from build123d import *

# Parameters (mm, degrees)
F0_W     = 96
F0_H     = 26
F0_R     = 4
F1_DEPTH = 2
F5_W     = 96
F5_H     = 26
F5_R     = 4
F6_DEPTH = 2
F4_W     = 96
F4_H     = 26
F4_R     = 4
F7_DEPTH = 2
F8_R     = 2


with BuildPart() as f1:
    # F0 (on Top) → F1 (new body)
    with BuildSketch(Plane.XY):
        with Locations((17.3164154523, 0.965568237)):
            Rectangle(F0_W, F0_H)
        with Locations((17.3164154523, 0.965568237)):
            Circle(F0_R, mode=Mode.SUBTRACT)
        with Locations((-18.6835845477, 0.965568237)):
            Circle(F0_R, mode=Mode.SUBTRACT)
        with Locations((53.3164154523, 0.965568237)):
            Circle(F0_R, mode=Mode.SUBTRACT)
    extrude(amount=F1_DEPTH)

    # F5 (on offset) → F6 (join)
    with BuildSketch(Plane.XZ.offset(12.034431763)):
        with Locations((17.3164154523, -11)):
            Rectangle(F5_W, F5_H)
        with Locations((-18.6835845477, -11)):
            Circle(F5_R, mode=Mode.SUBTRACT)
        with Locations((17.3164154523, -11)):
            Circle(F5_R, mode=Mode.SUBTRACT)
        with Locations((53.3164154523, -11)):
            Circle(F5_R, mode=Mode.SUBTRACT)
    extrude(amount=F6_DEPTH)

    # F4 (on offset) → F7 (join)
    with BuildSketch(Plane(origin=(0, 13.965568237, 0), x_dir=(-1, 0, 0), z_dir=(0, 1, 0))):
        with Locations((-17.3164154523, -11)):
            Rectangle(F4_W, F4_H)
        with Locations((-53.3164154523, -11)):
            Circle(F4_R, mode=Mode.SUBTRACT)
        with Locations((-17.3164154523, -11)):
            Circle(F4_R, mode=Mode.SUBTRACT)
        with Locations((18.6835845477, -11)):
            Circle(F4_R, mode=Mode.SUBTRACT)
    extrude(amount=F7_DEPTH)

    # F8
    f8_edges = [f1.edges().sort_by_distance(p)[0] for p in [
        (17.316415, -14.034432, 2),
        (17.316415, 15.965568, 2),
        (65.316415, 14.965568, -24),
        (65.316415, -13.034432, -24),
        (-30.683585, 14.965568, -24),
        (-30.683585, -13.034432, -24),
    ]]
    fillet(f8_edges, radius=F8_R)


solid = f1.part
Could you check a few things on this model? Use its own coordinates, in mm. A direction names the side the tool comes from. Round coordinates to 2 decimals unless told otherwise and drop trailing zeros. Write each loop counter-clockwise with the first axis right and the second up, starting at its lowest first coordinate (ties: lowest second). Pieces come first, ordered by that corner, then holes. Notation, with made-up numbers: (54.5, -4) -> (65.5, -4) arc R15 cw to (65.5, 6) -> close; hole circle Ø11 at (-39.5, -11). An arc over 180 degrees is marked (long way). Use a Markdown table: item, result.
1. If we section it at C-C (x = 15.5): List the corners of the cut face in (y, z) for me.
Answer key:
| item | result |
|---|---|
| outline | (-14.03, -24) -> (-12.03, -24) -> (-12.03, -14.56) -> (-14.03, -14.56) -> close; (-14.03, -7.44) -> (-12.03, -7.44) -> (-12.03, 0) -> (-2.6, 0) -> (-2.6, 2) -> (-12.03, 2) arc R2 ccw to (-14.03, 0) -> close; (4.53, 0) -> (13.97, 0) -> (13.97, -7.44) -> (15.97, -7.44) -> (15.97, 0) arc R2 ccw to (13.97, 2) -> (4.53, 2) -> close; (13.97, -24) -> (15.97, -24) -> (15.97, -14.56) -> (13.97, -14.56) -> close |
2. Which directions (+Z, -Z, +X, -X, +Y, -Y) give clear straight access to the entire face, cutting with the end or side of a thin tool? Please do faces 4 (the face through (17, -12.034, -17)), 5 (the face through (-17.8, 15, -14.9)).
Answer key:
| item | result |
|---|---|
| face 4 | -Z, +X, -X |
| face 5 | +Y, -Y |
3. If we section it at D-D (y = -4.75): List the corners of the cut face in (x, z) for me.
Answer key:
| item | result |
|---|---|
| outline | (-30.68, 0) -> (65.32, 0) -> (65.32, 2) -> (-30.68, 2) -> close |
4. For pin 1 Ø1.5 at (x, y) = (33.5, 6) entering from -Z; pin 2 Ø5 at (x, z) = (53.32, -11) entering from +Y, each with a flat end and sliding along its axis, tell me the tip position at first contact or that it passes through.
Answer key:
| item | result |
|---|---|
| pin 1 | stops at z = 0 |
| pin 2 | passes through |
5. If we section it at B-B (z = -11): State how many separate pieces and enclosed holes the cut face has, then the cut area to 3 significant figures.
Answer key:
| item | result |
|---|---|
| separate pieces | 8 |
| enclosed holes | 0 |
| area | 288 mm^2 |
6. Please list where these lines run through material, in increasing order: probe 1 along Y at (x, z) = (-1, -6); probe 2 along Z at (x, y) = (13, 0.75); probe 3 along X at (y, z) = (-1.5, 1).
Answer key:
| item | result |
|---|---|
| probe 1 | y = -14.03 to -12.03, 13.97 to 15.97 |
| probe 2 | z = 0 to 2 |
| probe 3 | x = -30.68 to -21.83, -15.53 to 14.17, 20.47 to 50.17, 56.47 to 65.32 |
7. If we section it at A-A (z = -16.25): List the corners of the cut face in (x, y) for me, then the cut area to 3 significant figures.
Answer key:
| item | result |
|---|---|
| outline | (-30.68, -14.03) -> (65.32, -14.03) -> (65.32, -12.03) -> (-30.68, -12.03) -> close; (-30.68, 13.97) -> (65.32, 13.97) -> (65.32, 15.97) -> (-30.68, 15.97) -> close |
| area | 384 mm^2 |
8. We'd pull the mould along X, two halves only. Please class faces 1 (the face through (65.316, 1, 1)), 2 (the face through (17, -13, -24)), 3 (the face through (49.32, -13.02, -10.82)): +X half, -X half, draft (parallel to the pull), parting line (faces both ways), or undercut.
Answer key:
| item | result |
|---|---|
| face 1 | +X half |
| face 2 | draft |
| face 3 | undercut |
